from build123d import *

# Parameters (mm, degrees)
F1_DEPTH = 6
F3_D     = 6.6
F4_SIZE  = 5


with BuildPart() as f1:
    # F0 (on Top) → F1 (new body)
    with BuildSketch(Plane.XY):
        Polygon((0, 85), (0, 0), (15.6104657799, 0), (20, 0), (40, 0), (40, 20), (20, 20), (20, 85), align=None)
    extrude(amount=F1_DEPTH)

    # F3 (through all)
    with Locations(Plane.XY.offset(6)):
        with Locations((10, 75), (10, 55), (10, 10), (30, 10), (10, 30)):
            Hole(F3_D / 2)

    # F4
    f4_edges = [f1.edges().sort_by_distance(p)[0] for p in [
        (20, 85, 3),
        (0, 85, 3),
        (40, 20, 3),
        (40, 0, 3),
        (0, 0, 3),
    ]]
    chamfer(f4_edges, length=F4_SIZE)


solid = f1.part
The model under review builds one solid part; all positions refer to its coordinate system, in mm. A direction names the side the tool comes from. Round coordinates to 2 decimals unless told otherwise and drop trailing zeros. Write each loop counter-clockwise with the first axis right and the second up, starting at its lowest first coordinate (ties: lowest second). Pieces come first, ordered by that corner, then holes. Notation, with made-up numbers: (85.25, 57.5) -> (139.25, 57.5) arc R9 ccw to (139.25, 71.5) -> close; hole circle Ø10 at (46, 77). An arc over 180 degrees is marked (long way). Answer as a JSON object with one key per item and string values.
1. Clearance check with flat-ended pins moving along their axes: pin 1 (7.5 mm diameter, centred on x = 30, y = 10, fed in from -Z); pin 2 (3 mm diameter, centred on x = 25.5, z = 4.5, fed in from +Y). State where each tip first meets the part, or that it passes through.
Results found:
{"pin 1": "stops at z = 0", "pin 2": "stops at y = 20"}
2. To check wall thickness, follow line 1 along Y through (x, z) = (10, 1.35); line 2 along X through (y, z) = (65, 2.4). State the ranges of each line that lie inside material, in increasing order.
Results found:
{"line 1": "y = 0 to 6.7, 13.3 to 26.7, 33.3 to 51.7, 58.3 to 71.7, 78.3 to 85", "line 2": "x = 0 to 20"}
3. We need section C-C on z = 3.5. State the section outline as (x, y) points, and give its area (3 significant figures).
Results found:
{"outline": "(0, 5) -> (5, 0) -> (35, 0) -> (40, 5) -> (40, 15) -> (35, 20) -> (20, 20) -> (20, 80) -> (15, 85) -> (5, 85) -> (0, 80) -> close; hole circle Ø6.6 at (10, 10); hole circle Ø6.6 at (10, 30); hole circle Ø6.6 at (10, 55); hole circle Ø6.6 at (10, 75); hole circle Ø6.6 at (30, 10)", "area": "1,870 mm^2"}
4. Machinability: for faces 5 (the face through (38, 3, 3)), 6 (the face through (20, 50, 3)), which of the approach directions +Z, -Z, +X, -X, +Y, -Y give a long, thin tool a straight path to every point of the face, cutting with its end or side? Answer none if there is none.
Results found:
{"face 5": "+Z, -Z, +X, -Y", "face 6": "+Z, -Z, +X, +Y"}
5. We need section A-A on y = 10. State the section outline as (x, z) points.
Results found:
{"outline": "(0, 0) -> (6.7, 0) -> (6.7, 6) -> (0, 6) -> close; (13.3, 0) -> (26.7, 0) -> (26.7, 6) -> (13.3, 6) -> close; (33.3, 0) -> (40, 0) -> (40, 6) -> (33.3, 6) -> close"}
6. We need section D-D on y = 30. State the section outline as (x, z) points.
Results found:
{"outline": "(0, 0) -> (6.7, 0) -> (6.7, 6) -> (0, 6) -> close; (13.3, 0) -> (20, 0) -> (20, 6) -> (13.3, 6) -> close"}
7. We need section B-B on x = 10. State the section outline as (y, z) points, and give its area (3 significant figures).
Results found:
{"outline": "(0, 0) -> (6.7, 0) -> (6.7, 6) -> (0, 6) -> close; (13.3, 0) -> (26.7, 0) -> (26.7, 6) -> (13.3, 6) -> close; (33.3, 0) -> (51.7, 0) -> (51.7, 6) -> (33.3, 6) -> close; (58.3, 0) -> (71.7, 0) -> (71.7, 6) -> (58.3, 6) -> close; (78.3, 0) -> (85, 0) -> (85, 6) -> (78.3, 6) -> close", "area": "352 mm^2"}
8. The part is to be moulded in two halves that separate along X. For faces 1 (the face through (3, 83, 3)), 2 (the face through (20, 0, 3)), 3 (the face through (12.619, 7.992, 2.958)), 4 (the face through (10.43, 58.27, 2.96)), say which applies: pulls with the +X half, pulls with the -X half, needs draft (parallel to the pull), parting line crosses it, or undercut.
Results found:
{"face 1": "pulls with the -X half", "face 2": "needs draft", "face 3": "undercut", "face 4": "undercut"}
